```python
from build123d import *

# Parameters (mm, degrees)
SKETCH3_W            = 200
SKETCH3_H            = 199.898
BOSS_EXTRUDE2_DEPTH  = 3
SKETCH9_W            = 3
SKETCH9_H            = 80
BOSS_EXTRUDE3_DEPTH  = 80
SKETCH10_W           = 3
SKETCH10_H           = 80
BOSS_EXTRUDE4_DEPTH  = 80
SKETCH11_W           = 200
SKETCH11_H           = 3
BOSS_EXTRUDE6_DEPTH  = 40
SKETCH23_R           = 6
CUT_EXTRUDE5_DEPTH   = 228.956
BOSS_EXTRUDE8_DEPTH  = 3
BOSS_EXTRUDE9_DEPTH  = 3
SKETCH30_R           = 6
CUT_EXTRUDE6_DEPTH   = 225.25
SKETCH32_W           = 200
SKETCH32_H           = 3
BOSS_EXTRUDE12_DEPTH = 83


with BuildPart() as part:
    # Sketch3 → Boss-Extrude2 (new body)
    with BuildSketch(Plane(origin=(0, 0, 0), x_dir=(1, 0, 0), z_dir=(0, 1, 0))):
        Rectangle(SKETCH3_W, SKETCH3_H)
    extrude(amount=BOSS_EXTRUDE2_DEPTH)

    # Sketch9 → Boss-Extrude3 (add)
    with BuildSketch(Plane(origin=(0, 3, 0), x_dir=(1, 0, 0), z_dir=(0, 1, 0))):
        with Locations((-98.5, 59.949)):
            Rectangle(SKETCH9_W, SKETCH9_H)
    extrude(amount=BOSS_EXTRUDE3_DEPTH)

    # Sketch10 → Boss-Extrude4 (add)
    with BuildSketch(Plane(origin=(0, 3, 0), x_dir=(1, 0, 0), z_dir=(0, 1, 0))):
        with Locations((98.5, 59.949)):
            Rectangle(SKETCH10_W, SKETCH10_H)
    extrude(amount=BOSS_EXTRUDE4_DEPTH)

    # Sketch11 → Boss-Extrude6 (add)
    with BuildSketch(Plane(origin=(0, 0, 0), x_dir=(1, 0, 0), z_dir=(0, 1, 0))):
        with Locations((0, -98.449)):
            Rectangle(SKETCH11_W, SKETCH11_H)
    extrude(amount=BOSS_EXTRUDE6_DEPTH)

    # Sketch23 → Cut-Extrude5 (cut)
    with BuildSketch(Plane.ZY.offset(100)):
        with Locations((-59.949, 33)):
            Circle(SKETCH23_R)
    extrude(amount=-CUT_EXTRUDE5_DEPTH, mode=Mode.SUBTRACT)

    # Sketch26 → Boss-Extrude8 (add)
    with BuildSketch(Plane.ZY.offset(100)):
        with BuildLine():
            Line((99.949, 0), (99.949, 40))
            Line((99.949, 40), (96.949, 40))
            ThreePointArc((96.949, 40), (34.223384101, 49.873771039), (-19.949, 83))
            Line((-19.949, 83), (-99.949, 83))
            Line((-99.949, 83), (-99.949, 0))
            Line((-99.949, 0), (99.949, 0))
        make_face()
    extrude(amount=-BOSS_EXTRUDE8_DEPTH)

    # Sketch29 → Boss-Extrude9 (add)
    with BuildSketch(Plane(origin=(100, 0, 0), x_dir=(0, 0, -1), z_dir=(1, 0, 0))):
        with BuildLine():
            ThreePointArc((19.949, 83), (-34.223384101, 49.873771039), (-96.949, 40))
            Line((-96.949, 40), (-96.949, 3))
            Line((-96.949, 3), (19.949, 3))
            Line((19.949, 3), (19.949, 83))
        make_face()
    extrude(amount=-BOSS_EXTRUDE9_DEPTH)

    # Sketch30 → Cut-Extrude6 (cut)
    with BuildSketch(Plane(origin=(100, 0, 0), x_dir=(0, 0, -1), z_dir=(1, 0, 0))):
        with Locations((59.949, 33)):
            Circle(SKETCH30_R)
    extrude(amount=-CUT_EXTRUDE6_DEPTH, mode=Mode.SUBTRACT)

    # Sketch32 → Boss-Extrude12 (add)
    with BuildSketch(Plane(origin=(0, 0, 0), x_dir=(1, 0, 0), z_dir=(0, 1, 0))):
        with Locations((0, 98.449)):
            Rectangle(SKETCH32_W, SKETCH32_H)
    extrude(amount=BOSS_EXTRUDE12_DEPTH)


solid = part.part
```
Verification items for the finished model (mm, model axes). A direction names the side the tool comes from. Round coordinates to 2 decimals unless told otherwise and drop trailing zeros. Order: outer loops, then holes, each group sorted by start corner. A loop starts at its lowest first (then second) coordinate and runs counter-clockwise, first axis right, second up.
1) Depth check by flat-ended pin: pin 1 (8 mm diameter, centred on x = -50, z = -70, fed in from -Y); pin 2 (3 mm diameter, centred on x = -58.5, y = 48, fed in from +Z); pin 3 (0.9 mm diameter, centred on x = -48, z = 98.5, fed in from +Y). Enter the tip coordinate at first touch or a pass-through.
Geometry says:
pin 1: stops at y = 0
pin 2: stops at z = -96.95
pin 3: stops at y = 40
2) Cross-section at D-D, the plane y = 13.5. Record the cut outline in (x, z).
Geometry says:
outline: (-100, -99.95) - (100, -99.95) - (100, 99.95) - (-100, 99.95) - close; hole (-97, -96.95) - (97, -96.95) - (97, 96.95) - (-97, 96.95) - close
3) Cross-section at C-C, the plane x = 10.5. Record the cut outline in (y, z).
Geometry says:
outline: (0, -99.95) - (83, -99.95) - (83, -96.95) - (3, -96.95) - (3, 96.95) - (40, 96.95) - (40, 99.95) - (0, 99.95) - close
4) Cross-section at A-A, the plane z = -57.5. Record the cut outline in (x, y), plus the area to 3 significant figures.
Geometry says:
outline: (-100, 0) - (100, 0) - (100, 27.52) - (97, 27.52) - (97, 3) - (-97, 3) - (-97, 27.52) - (-100, 27.52) - close; (-100, 38.48) - (-97, 38.48) - (-97, 83) - (-100, 83) - close; (97, 38.48) - (100, 38.48) - (100, 83) - (97, 83) - close
area: 1,010 mm2
5) Tool access check on faces 4 (the flat face through (97, 35, -20)), 5 (the flat face through (-100, 32, -21)). Record the directions out of +Z, -Z, +X, -X, +Y, -Y that give a thin tool (end or side, any length) a straight path to the whole face; none if there is none.
Geometry says:
face 4: +Y
face 5: +Z, -Z, -X, +Y, -Y
6) Material ranges on line 1 (Z direction, x = 98, y = 33); line 2 (X direction, y = 48, z = -51); line 3 (Z direction, x = 24.5, y = 35), recorded low to high.
Geometry says:
line 1: z = -99.95 to -65.95, -53.95 to 99.95
line 2: x = -100 to -97, 97 to 100
line 3: z = -99.95 to -96.95, 96.95 to 99.95
7) Cross-section at B-B, the plane y = 33. Record the cut outline in (x, z).
Geometry says:
outline: (-100, -99.95) - (100, -99.95) - (100, -65.95) - (97, -65.95) - (97, -96.95) - (-97, -96.95) - (-97, -65.95) - (-100, -65.95) - close; (-100, -53.95) - (-97, -53.95) - (-97, 96.95) - (97, 96.95) - (97, -53.95) - (100, -53.95) - (100, 99.95) - (-100, 99.95) - close
8) Draft check along Y on faces 1 (the cylindrical face through (-98.52, 49.57, 35.06)), 2 (the flat face through (-1, 0, -1)), 3 (the cylindrical face through (98.479, 27.143, -61.25)). Enter one of: +Y half, -Y half, draft (parallel to the pull), parting line (faces both ways), or undercut.
Geometry says:
face 1: +Y half
face 2: -Y half
face 3: undercut
